```python
from build123d import *

# Parameters (mm, degrees)
BOSS_EXTRUDE1_DEPTH = 5


with BuildPart() as part:
    # Sketch2 → Boss-Extrude1 (new body)
    with BuildSketch(Plane.XY):
        with BuildLine():
            Line((0, 5.5), (50, 5.5))
            ThreePointArc((50, 5.5), (55.5, 0), (50, -5.5))
            Line((50, -5.5), (0, -5.5))
            ThreePointArc((0, -5.5), (-5.5, 0), (0, 5.5))
        make_face()
        with BuildLine():
            ThreePointArc((50, -2.5), (52.5, 0), (50, 2.5))
            Line((50, 2.5), (0, 2.5))
            ThreePointArc((0, 2.5), (-2.5, 0), (0, -2.5))
            Line((0, -2.5), (50, -2.5))
        make_face(mode=Mode.SUBTRACT)
    extrude(amount=BOSS_EXTRUDE1_DEPTH)


solid = part.part
```
Here's how the part is built. I have some questions about the finished solid (model axes, mm). A direction names the side the tool comes from. Round coordinates to 2 decimals unless told otherwise and drop trailing zeros. Write each loop counter-clockwise with the first axis right and the second up, starting at its lowest first coordinate (ties: lowest second). Pieces come first, ordered by that corner, then holes.
Q1. Which directions (+Z, -Z, +X, -X, +Y, -Y) give clear straight access to the entire face, cutting with the end or side of a thin tool? Please do faces 4 (the flat face through (25, 5.5, 2)), 5 (the flat face through (25, 2.5, 2)).
Q2. If we section it at B-B on z = 0.95: Write out the boundary of the cut face in (x, y).
Q3. Please list where these lines run through material, in increasing order: probe 1 along Y at (x, z) = (5, 2.95); probe 2 along X at (y, z) = (0.25, 3.4); probe 3 along Y at (x, z) = (-1, 1.1).
Q4. If we mould it in two halves opening along Y, with no side actions, what happens to faces 1 (the flat face through (25, -2.5, 2)), 2 (the flat face through (25, -5.5, 2)), 3 (the flat face through (25, 3, 0))? For each: +Y half, -Y half, draft (parallel to the pull), parting line (faces both ways), or undercut.
Q5. If we section it at A-A on x = 37.5: Write out the boundary of the cut face in (y, z).
Q6. If we section it at C-C on y = 0: Write out the boundary of the cut face in (x, z).
Q7. Will this pin go through, and if not, where does the flat tip stop? P1, Ø3, axis at y = 1.5, z = 3, coming from the -X side.
Answer below:
1. face 4: +Z, -Z, +X, -X, +Y
1. face 5: +Z, -Z
2. outline: (0, -5.5) - (50, -5.5) arc R5.5 ccw to (50, 5.5) - (0, 5.5) arc R5.5 ccw to start; hole (0, -2.5) - (50, -2.5) arc R2.5 ccw to (50, 2.5) - (0, 2.5) arc R2.5 ccw to start
3. probe 1: y = -5.5 to -2.5, 2.5 to 5.5
3. probe 2: x = -5.49 to -2.49, 52.49 to 55.49
3. probe 3: y = -5.41 to -2.29, 2.29 to 5.41
4. face 1: undercut
4. face 2: -Y half
4. face 3: draft
5. outline: (-5.5, 0) - (-2.5, 0) - (-2.5, 5) - (-5.5, 5) - close; (2.5, 0) - (5.5, 0) - (5.5, 5) - (2.5, 5) - close
6. outline: (-5.5, 0) - (-2.5, 0) - (-2.5, 5) - (-5.5, 5) - close; (52.5, 0) - (55.5, 0) - (55.5, 5) - (52.5, 5) - close
7. P1: stops at x = -5.5
